For this review, take the finished solid that the model builds, in its own axes (mm). Face numbers are marked on the shaded views. Round coordinates to 2 decimals unless told otherwise and drop trailing zeros. Order: outer loops, then holes, each group sorted by start corner. A loop starts at its lowest first (then second) coordinate and runs counter-clockwise, first axis right, second up. Notation, with made-up numbers: (18, -5.5) -> (75, -5.5) arc R16 cw to (75, 9.5) -> close; hole circle Ø5 at (18.25, 30). An arc over 180 degrees is marked (long way). Use a Markdown table: item, result. Add a question column.
1) Wall thickness on line 1 along X through (y, z) = (1.45, -0.15); line 2 along X through (y, z) = (1.35, -0.2); line 3 along X through (y, z) = (-1.5, -0.25): over which ranges is each line inside the solid? List them lowest first. Write a range as [from, to].
2) Consider section B-B (z = -0.3). State the section outline as (x, y) points.
3) Draft analysis for pull direction Y (two halves, no side actions). For the marked faces 1, 2 and 3, state which applies: pulls with the +Y half, pulls with the -Y half, needs draft (parallel to the pull), parting line crosses it, or undercut.
4) Consider section C-C (x = 0). State the section outline as (y, z) points, plus the area to 3 significant figures.
5) Consider section D-D (y = 0.85). State the section outline as (x, z) points, plus the area to 3 significant figures.
6) Consider section A-A (y = -0.5). State the section outline as (x, z) points.
```python
from build123d import *

# Parameters (mm, degrees)
BODY_DEPTH = 0.4


with BuildPart() as part:
    # Sketch1 → Body (new body)
    with BuildSketch(Plane.XY):
        with BuildLine():
            Line((0.517084333, 1.59142194), (0.386271243, 1.188820645))
            ThreePointArc((0.386271243, 1.188820645), (0, 1.25), (-0.386271243, 1.188820645))
            Line((-0.386271243, 1.188820645), (-0.517084333, 1.59142194))
            ThreePointArc((-0.517084333, 1.59142194), (-0.690418116, 1.777032794), (-0.944001516, 1.763196285))
            ThreePointArc((-0.944001516, 1.763196285), (-1.414213562, 1.414213562), (-1.763196285, 0.944001516))
            ThreePointArc((-1.763196285, 0.944001516), (-1.777032794, 0.690418116), (-1.59142194, 0.517084333))
            Line((-1.59142194, 0.517084333), (-1.188820645, 0.386271243))
            ThreePointArc((-1.188820645, 0.386271243), (-1.244897296, -0.112830506), (-1.1, -0.593717104))
            Line((-1.1, -0.593717104), (-1.526646887, -2.081611619))
            ThreePointArc((-1.526646887, -2.081611619), (-1.732937183, -2.287471145), (-2.016694884, -2.22102268))
            ThreePointArc((-2.016694884, -2.22102268), (0, 3), (2.016694884, -2.22102268))
            ThreePointArc((2.016694884, -2.22102268), (1.732937183, -2.287471145), (1.526646887, -2.081611619))
            Line((1.526646887, -2.081611619), (1.1, -0.593717104))
            ThreePointArc((1.1, -0.593717104), (1.244897296, -0.112830506), (1.188820645, 0.386271243))
            Line((1.188820645, 0.386271243), (1.59142194, 0.517084333))
            ThreePointArc((1.59142194, 0.517084333), (1.777032794, 0.690418116), (1.763196285, 0.944001516))
            ThreePointArc((1.763196285, 0.944001516), (1.414213562, 1.414213562), (0.944001516, 1.763196285))
            ThreePointArc((0.944001516, 1.763196285), (0.690418116, 1.777032794), (0.517084333, 1.59142194))
        make_face()
    extrude(amount=-BODY_DEPTH)


solid = part.part
```
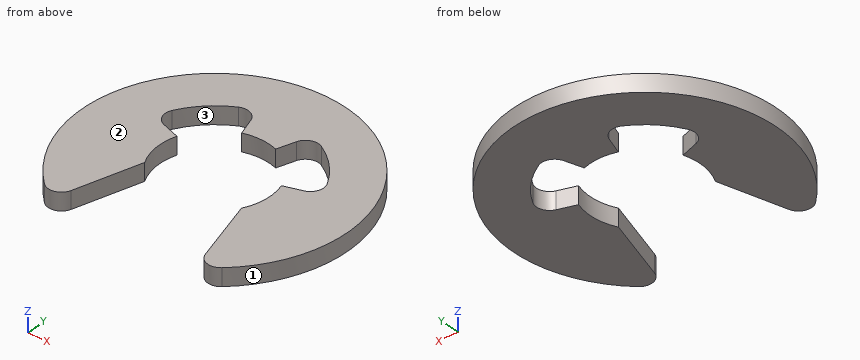
Results list:
| question | item | result |
|---|---|---|
| 1 | line 1 | [-2.63, -1.38], [-0.47, 0.47], [1.38, 2.63] |
| 1 | line 2 | [-2.68, -1.48], [-0.44, 0.44], [1.48, 2.68] |
| 1 | line 3 | [-2.6, -1.36], [1.36, 2.6] |
| 2 | outline | (-2.02, -2.22) arc R0.3 ccw to (-1.53, -2.08) -> (-1.1, -0.59) arc R1.25 cw to (-1.19, 0.39) -> (-1.59, 0.52) arc R0.3 cw to (-1.76, 0.94) arc R2 cw to (-0.94, 1.76) arc R0.3 cw to (-0.52, 1.59) -> (-0.39, 1.19) arc R1.25 cw to (0.39, 1.19) -> (0.52, 1.59) arc R0.3 cw to (0.94, 1.76) arc R2 cw to (1.76, 0.94) arc R0.3 cw to (1.59, 0.52) -> (1.19, 0.39) arc R1.25 cw to (1.1, -0.59) -> (1.53, -2.08) arc R0.3 ccw to (2.02, -2.22) arc R3 ccw (long way) to start |
| 3 | face 1 | parting line crosses it |
| 3 | face 2 | needs draft |
| 3 | face 3 | undercut |
| 4 | outline | (1.25, -0.4) -> (3, -0.4) -> (3, 0) -> (1.25, 0) -> close |
| 4 | area | 0.700 mm2 |
| 5 | outline | (-2.88, -0.4) -> (-1.79, -0.4) -> (-1.79, 0) -> (-2.88, 0) -> close; (1.79, -0.4) -> (2.88, -0.4) -> (2.88, 0) -> (1.79, 0) -> close |
| 5 | area | 0.866 mm2 |
| 6 | outline | (-2.96, -0.4) -> (-1.15, -0.4) -> (-1.15, 0) -> (-2.96, 0) -> close; (1.15, -0.4) -> (2.96, -0.4) -> (2.96, 0) -> (1.15, 0) -> close |
